Model file for the job. Use its own axes, mm. Face numbers are marked on the shaded views. A direction names the side the tool comes from. Round coordinates to 2 decimals unless told otherwise and drop trailing zeros. Loops run counter-clockwise (first coordinate to the right, second up) from the corner with the lowest first, then second, coordinate; pieces in that order, holes last. Notation, with made-up numbers: M 11.25,52 L 62.25,52 A30 cw 62.25,84 Z; hole C 13.25,35.25 d2. An arc over 180 degrees is marked long. Answer in a Markdown table with one row per item.
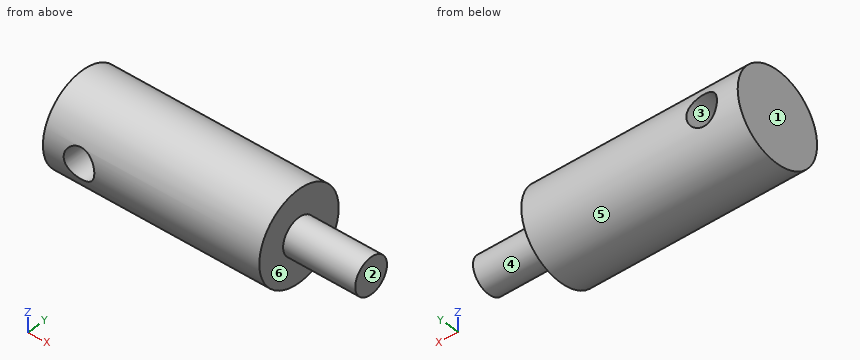
Autodesk Inventor part; units mm, degrees
ref_plane "YZ Plane" through (0, 0, 0) normal (1, 0, 0) x (0, 1, 0)
ref_plane "XZ Plane" through (0, 0, 0) normal (0, 1, 0) x (-1, 0, 0)
ref_plane "XY Plane" through (0, 0, 0) normal (0, 0, 1) x (1, 0, 0)
sketch "Boceto3" plane through (0, 0, 0) normal (0, 0, 1) x (1, 0, 0)
  line L0 (0, 0) -> (0, 12.5)
  line L1 (0, 12.5) -> (60, 12.5)
  line L2 (60, 12.5) -> (60, 5)
  line L3 (60, 5) -> (80, 5)
  line L4 (80, 5) -> (80, 0)
  line L5 (80, 0) -> (0, 0)
  dimension "d16" = 12.5
  dimension "d17" = 60
  dimension "d18" = 20
  dimension "d19" = 5
revolve "Revolución1" add sketch "Boceto3" angle 360 about axis through (80, 0, 0) along (-1, 0, 0)
sketch "Boceto4" plane through (0, 0, 0) normal (0, 1, 0) x (-1, 0, 0)
  circle A0 centre (-10, 0) radius 4.25
  line L0 (-60, 12.5) -> (-60, -12.5)
  point P0 (0, 0)
  dimension "d21" = 8.5
  dimension "d22" = 50
extrude "Extrusión3" cut sketch "Boceto4" along normal through all both and the other way through all
thread "Rosca3"
thread "Rosca4"
properties part number "brazos_planetarios1" material "Nilón 6/6"
1. Tool access for the marked faces 5 and 6: list every direction of +Z, -Z, +X, -X, +Y, -Y with a clear straight run to the whole face (end or side of a thin tool).
Verdict:
| item | result |
|---|---|
| face 5 | +X, -X |
| face 6 | +X |
2. Saw through at D-D (x = 35). Write the cut outline in (y, z).
Verdict:
| item | result |
|---|---|
| outline | C 0,0 d25 |
3. Saw through at A-A (z = 0). Write the cut outline in (x, y), and give its area (3 significant figures).
Verdict:
| item | result |
|---|---|
| outline | M 0,-12.5 L 5.75,-12.5 L 5.75,12.5 L 0,12.5 Z; M 14.25,-12.5 L 60,-12.5 L 60,-5 L 80,-5 L 80,5 L 60,5 L 60,12.5 L 14.25,12.5 Z |
| area | 1,490 mm² |
4. Pin check, flat tips, straight feed: pin 1 (1.5 mm diameter, centred on x = 48, y = 2.5, fed in from +Z); pin 2 (4 mm diameter, centred on x = 20.5, z = -2.5, fed in from -Y); pin 3 (5 mm diameter, centred on x = 63.5, z = 2, fed in from -Y). Stop position of each tip, or through.
Verdict:
| item | result |
|---|---|
| pin 1 | stops at z = 12.38 |
| pin 2 | stops at y = -12.49 |
| pin 3 | stops at y = -5 |
5. Saw through at C-C (x = 10). Write the cut outline in (y, z), and give its area (3 significant figures).
Verdict:
| item | result |
|---|---|
| outline | M -11.76,-4.25 A12.5 ccw 11.76,-4.25 Z; M -11.76,4.25 L 11.76,4.25 A12.5 ccw Z |
| area | 283 mm² |
6. Saw through at B-B (y = 0). Write the cut outline in (x, z).
Verdict:
| item | result |
|---|---|
| outline | M 0,-12.5 L 60,-12.5 L 60,-5 L 80,-5 L 80,5 L 60,5 L 60,12.5 L 0,12.5 Z; hole C 10,0 d8.5 |
7. Mould opens along X. For the marked faces 1, 2, 3 and 4 say: +X half, -X half, draft (parallel to the pull), parting line (faces both ways), or undercut.
Verdict:
| item | result |
|---|---|
| face 1 | -X half |
| face 2 | +X half |
| face 3 | undercut |
| face 4 | draft |
8. Wall check: probe 1 along X at (y, z) = (-5.5, 0); probe 2 along X at (y, z) = (-2.5, 0); probe 3 along Y at (x, z) = (35.5, 0.25). Give the ranges that are in metal, low to high.
Verdict:
| item | result |
|---|---|
| probe 1 | x = 0 to 5.75, 14.25 to 60 |
| probe 2 | x = 0 to 5.75, 14.25 to 80 |
| probe 3 | y = -12.5 to 12.5 |
